```python
from build123d import *

# Parameters (mm, degrees)
BOSS_EXTRUDE1_DEPTH = 10
SKETCH2_R           = 8
CUT_EXTRUDE1_DEPTH  = 5
FILLET1_R           = 10
SKETCH4_R           = 2
CUT_EXTRUDE3_DEPTH  = 22
SKETCH5_R           = 2
CUT_EXTRUDE4_DEPTH  = 23
SKETCH6_R           = 5
CUT_EXTRUDE5_DEPTH  = 10
SKETCH8_W           = 16
SKETCH8_H           = 34
CUT_EXTRUDE7_DEPTH  = 10


with BuildPart() as part:
    # Sketch1 → Boss-Extrude1 (new body)
    with BuildSketch(Plane.XY):
        Polygon((-37.625, -24), (18.375, -24), (18.375, -12), (8.375, -12), (8.375, 53), (-27.625, 53), (-27.625, -12), (-37.625, -12), align=None)
    extrude(amount=BOSS_EXTRUDE1_DEPTH)

    # Sketch2 → Cut-Extrude1 (cut)
    with BuildSketch(Plane.XY.offset(10)):
        with Locations((-9.625, 38)):
            Circle(SKETCH2_R)
    extrude(amount=-CUT_EXTRUDE1_DEPTH, mode=Mode.SUBTRACT)

    # Fillet1
    fillet1_edges = [part.edges().sort_by_distance(p)[0] for p in [
        (8.375, 53, 5),
        (-27.625, 53, 5),
    ]]
    fillet(fillet1_edges, radius=FILLET1_R)

    # Sketch4 → Cut-Extrude3 (cut)
    with BuildSketch(Plane(origin=(0, -12, 0), x_dir=(1, 0, 0), z_dir=(0, 1, 0))):
        with Locations(Location((13.375, -5, 0), (0, 0, 180))):
            Circle(SKETCH4_R)
    extrude(amount=-CUT_EXTRUDE3_DEPTH, mode=Mode.SUBTRACT)

    # Sketch5 → Cut-Extrude4 (cut)
    with BuildSketch(Plane(origin=(0, -12, 0), x_dir=(1, 0, 0), z_dir=(0, 1, 0))):
        with Locations(Location((-32.625, -5, 0), (0, 0, 270))):
            Circle(SKETCH5_R)
    extrude(amount=-CUT_EXTRUDE4_DEPTH, mode=Mode.SUBTRACT)

    # Sketch6 → Cut-Extrude5 (cut)
    with BuildSketch(Plane.XY.offset(5)):
        with Locations((-9.625, 38)):
            Circle(SKETCH6_R)
    extrude(amount=-CUT_EXTRUDE5_DEPTH, mode=Mode.SUBTRACT)

    # Sketch8 → Cut-Extrude7 (cut)
    with BuildSketch(Plane.XY.offset(10)):
        with Locations((-9.625, 5)):
            Rectangle(SKETCH8_W, SKETCH8_H)
    extrude(amount=-CUT_EXTRUDE7_DEPTH, mode=Mode.SUBTRACT)


solid = part.part
```
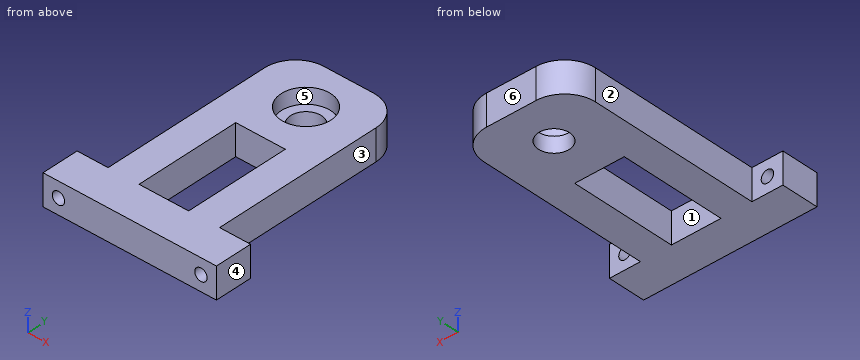
Input: part model. Units: mm. Frame: model coordinates. Face numbers are marked on the shaded views. A direction names the side the tool comes from. Give positions to 0.01 mm unless a question says otherwise; leave off trailing zeros. Order: outer loops, then holes, each group sorted by start corner. A loop starts at its lowest first (then second) coordinate and runs counter-clockwise, first axis right, second up. Notation, with made-up numbers: M 38.5,-31.75 L 62.5,-31.75 A26 ccw 62.5,-14.75 Z; hole C 78,9 d5. An arc over 180 degrees is marked long. Return JSON: item names as keys, results as strings.
Item 1: First-contact query: P1, Ø5, axis at y = -1.5, z = 2.5, coming from the -X side (3 decimals); P2, Ø21, axis at x = -9.625, y = 38, coming from the +Z side; P3, Ø3, axis at y = -2, z = 3.5, coming from the +X side (3 decimals); P4, Ø3, axis at x = -32, z = 8, coming from the +Y side. Flat tips, straight axial feed; report the tip coordinate or a pass-through.
Solutions:
{"P1": "x = -27.625", "P2": "z = 10", "P3": "x = 8.375", "P4": "y = -12"}
Item 2: Ray query, probe 1 along X at (y, z) = (-2.5, 9.75) (3 decimals); probe 2 along Y at (x, z) = (-7, 6.75); probe 3 along Y at (x, z) = (-5, 8.5). Return the intervals inside material, ascending.
Solutions:
{"probe 1": "-27.625 to -17.625, -1.625 to 8.375", "probe 2": "-24 to -12, 22 to 30.44, 45.56 to 53", "probe 3": "-24 to -12, 22 to 31.47, 44.53 to 53"}
Item 3: Cut plane B-B (y = 12). Return loops of the section in (x, z) (3 decimals).
Solutions:
{"outline": "M -27.625,0 L -17.625,0 L -17.625,10 L -27.625,10 Z; M -1.625,0 L 8.375,0 L 8.375,10 L -1.625,10 Z"}
Item 4: Cut plane A-A (y = 38). Return loops of the section in (x, z) (3 decimals), then the cut area to 3 significant figures.
Solutions:
{"outline": "M -27.625,0 L -14.625,0 L -14.625,5 L -17.625,5 L -17.625,10 L -27.625,10 Z; M -4.625,0 L 8.375,0 L 8.375,10 L -1.625,10 L -1.625,5 L -4.625,5 Z", "area": "230 mm^2"}
Item 5: Access query for the marked faces 1, 2 and 3. Directions: +Z, -Z, +X, -X, +Y, -Y. A direction counts if a zero-diameter tool reaches every point of the face in a straight line with its end or side. Return the directions, or none.
Solutions:
{"face 1": "+Z, -Z", "face 2": "+Z, -Z, -X, +Y", "face 3": "+Z, -Z, +X, +Y"}
Item 6: Pull-direction query (X, two-part tool) for the marked faces 4, 5 and 6; classes: +X half, -X half, draft (parallel to the pull), parting line (faces both ways), or undercut.
Solutions:
{"face 4": "+X half", "face 5": "undercut", "face 6": "draft"}
Item 7: Cut plane C-C (x = -25). Return loops of the section in (y, z).
Solutions:
{"outline": "M -24,0 L 49.75,0 L 49.75,10 L -24,10 Z"}
Item 8: Cut plane D-D (y = 25). Return loops of the section in (x, z) (3 decimals), then the cut area to 3 significant figures.
Solutions:
{"outline": "M -27.625,0 L 8.375,0 L 8.375,10 L -27.625,10 Z", "area": "360 mm^2"}
